Source: CAD feature listing. Evaluate the final solid. Frame: model axes, mm. Face numbers are marked on the shaded views. A direction names the side the tool comes from. Round coordinates to 2 decimals unless told otherwise and drop trailing zeros. Write each loop counter-clockwise with the first axis right and the second up, starting at its lowest first coordinate (ties: lowest second). Pieces come first, ordered by that corner, then holes. Notation, with made-up numbers: (55, 89) -> (87, 89) arc R17 ccw to (87, 119) -> close; hole circle Ø11 at (28.5, 1). An arc over 180 degrees is marked (long way). Put each result on its own line as item: value.
```python
from build123d import *

# Parameters (mm, degrees)
BOSS_EXTRUDE1_DEPTH = 3.5
SKETCH16_OUTSIDE_W  = 57.702
SKETCH16_OUTSIDE_H  = 58.94
SKETCH16_OUTSIDE_R  = 4
CUT_EXTRUDE7_DEPTH  = 12.718930555
CUT_EXTRUDE7_DRAFT  = -60
CHAMFER1_SIZE       = 0.6


with BuildPart() as part:
    # Sketch1 → Revolve1 (revolve)
    with BuildSketch(Plane(origin=(0, 0, 0), x_dir=(0, 0, -1), z_dir=(1, 0, 0))):
        Polygon((3.5, 2.5), (13.5, 2.5), (13.5, 0), (0, 0), (0, 4), (3.5, 4), align=None)
    revolve(axis=Axis((0, 0, -13.5), (0, 0, 1)))

    # Sketch2 → Boss-Extrude1 (add)
    with BuildSketch(Plane.XY):
        Polygon((4, 2.309401077), (0, 4.618802154), (-4, 2.309401077), (-4, -2.309401077), (0, -4.618802154), (4, -2.309401077), align=None)
    extrude(amount=-BOSS_EXTRUDE1_DEPTH)

    # Cut-Extrude2: read off the stored shape, not the designer's step
    # Cut-Extrude2 outline → Cut-Extrude2 (revolve, cut)
    with BuildSketch(Plane.XZ):
        Polygon((4.618802154, 2.09e-07), (3.999999819, 2.09e-07), (4.618802154, -0.35726559), align=None)
    revolve(axis=Axis((0, 0, 0), (0, 0, 1)), mode=Mode.SUBTRACT)

    # Cut-Extrude2 2 outline → Cut-Extrude2 2 (revolve, cut)
    with BuildSketch(Plane.XZ):
        Polygon((4.618802154, 2.09e-07), (3.999999819, 2.09e-07), (4.618802154, -0.35726559), align=None)
    revolve(axis=Axis((0, 0, 0), (0, 0, 1)), mode=Mode.SUBTRACT)


with BuildPart() as cut_extrude7_tool:
    # Sketch16 outside → Cut-Extrude7 (with draft: the straight prism first)
    with BuildSketch(Plane(origin=(0, 0, -3.5), x_dir=(-1, 0, 0), z_dir=(0, 0, -1))):
        Rectangle(SKETCH16_OUTSIDE_W, SKETCH16_OUTSIDE_H)
        Circle(SKETCH16_OUTSIDE_R, mode=Mode.SUBTRACT)
    extrude(amount=-CUT_EXTRUDE7_DEPTH)
    # Cut-Extrude7: the draft: its side faces are tilted about the plane it starts from
    cut_extrude7_sides = [cut_extrude7_tool.faces().sort_by_distance(p)[0] for p in [
        (0, -29.47, 2.859465277),
        (-28.851, 0, 2.859465277),
        (0, 29.47, 2.859465277),
        (28.851, 0, 2.859465277),
        (4, 0, 2.859465277),
    ]]
    draft(cut_extrude7_sides, Plane(origin=(0, 0, -3.5), x_dir=(-1, 0, 0), z_dir=(0, 0, -1)), CUT_EXTRUDE7_DRAFT)


with BuildPart() as part_1:
    add(part.part)

    # Cut-Extrude7: cut by cut_extrude7_tool
    add(cut_extrude7_tool.part, mode=Mode.SUBTRACT)

    # Chamfer1
    chamfer1_edges = [part_1.edges().sort_by_distance(p)[0] for p in [
        (0, -2.5, -13.5),
    ]]
    chamfer(chamfer1_edges, length=CHAMFER1_SIZE)


solid = part_1.part
```
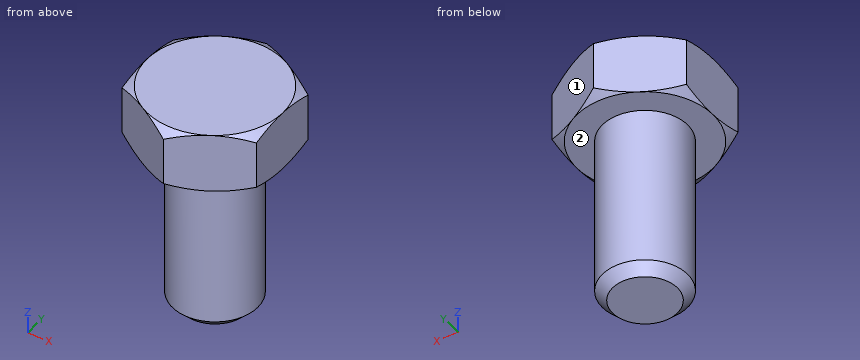
Q1. Pin query (flat end, axial travel): pin 1 (2 mm diameter, centred on x = 1.5, z = -4, fed in from +Y); pin 2 (5 mm diameter, centred on y = -1.5, z = -12, fed in from -X); pin 3 (1 mm diameter, centred on x = 2.5, z = -8.5, fed in from +Y). Return the tip coordinate at first contact, or that it passes through.
Ans:
pin 1: stops at y = 4.19
pin 2: stops at x = -2.5
pin 3: stops at y = 1.5
Q2. Reachability of the marked faces 1 and 2 from +Z, -Z, +X, -X, +Y, -Y: full face, straight path, thin tool, end or side. Return the list, or none.
Ans:
face 1: +Z, -Z, +X, +Y
face 2: -Z
Q3. Material intervals for line 1 (X direction, y = 0, z = -11.5); line 2 (Z direction, x = -2, y = 3.25); line 3 (Y direction, x = 1.5, z = -8), sorted ascending. Write a range as [from, to].
Ans:
line 1: x = [-2.5, 2.5]
line 2: z = [-3.5, 0]
line 3: y = [-2, 2]
Q4. Cut plane A-A on z = -10.75. Output: boundary loops of the cut face in (x, y), and give its area (3 significant figures).
Ans:
outline: circle Ø5 at (0, 0)
area: 19.6 mm^2
